Here's how the part is built. I have some questions about the finished solid (model axes, mm). A direction names the side the tool comes from. Give positions to 0.01 mm unless a question says otherwise; leave off trailing zeros. Loops run counter-clockwise (first coordinate to the right, second up) from the corner with the lowest first, then second, coordinate; pieces in that order, holes last. Notation, with made-up numbers: (-31, 32.25) - (-11, 32.25) arc R24 ccw to (-11, 69.25) - close; hole circle Ø5 at (-36, -25). An arc over 180 degrees is marked (long way). Put each result on its own line as item: value. Start each with the question number.
Autodesk Inventor part; units mm, degrees
ref_plane "YZ Plane" through (0, 0, 0) normal (1, 0, 0) x (0, 1, 0)
ref_plane "XZ Plane" through (0, 0, 0) normal (0, 1, 0) x (-1, 0, 0)
ref_plane "XY Plane" through (0, 0, 0) normal (0, 0, 1) x (1, 0, 0)
sketch "Sketch1" plane through (0, 0, 0) normal (0, 0, 1) x (1, 0, 0)
  line L0 (0, 12.6) -> (150, 12.6)
  arc A0 (150, -12.6) -> (150, 12.6) centre (150, 0) ccw
  line L1 (150, -12.6) -> (0, -12.6)
  arc A1 (0, 12.6) -> (0, -12.6) centre (0, 0) ccw
  circle A2 centre (0, 0) radius 7.5
  circle A3 centre (150, 0) radius 4.25
  dimension "d0" = 150
  dimension "d2" = 12.6
  dimension "d3" = 15
  dimension "d4" = 8.5
extrude "Extrusion1" add sketch "Sketch1" along normal blind 25
sketch "Sketch2" plane through (0, 0, 25) normal (0, 0, 1) x (1, 0, 0)
  circle A0 centre (0, 0) radius 7.5
  arc A1 (0, 12.6) -> (0, -12.6) centre (0, 0) ccw
  circle A2 centre (0, 0) radius 11
  dimension "d7" = 22
extrude "Extrusion2" cut sketch "Sketch2" against normal blind 7
sketch "Sketch4" plane through (0, 0, 25) normal (0, 0, 1) x (1, 0, 0)
  circle A0 centre (0, 0) radius 11
  circle A1 centre (20, 0) radius 1.75
  circle A2 centre (40, 0) radius 1.75
  dimension "d16" = 20
  dimension "d17" = 40
  dimension "d23" = 3.5
extrude "Extrusion3" cut sketch "Sketch4" against normal through all contours A1 | A2
sketch "Sketch5" plane through (0, 0, 25) normal (0, 0, 1) x (1, 0, 0)
  circle A0 centre (20, 0) radius 1.75
  circle A1 centre (40, 0) radius 1.75
  circle A2 centre (40, 0) radius 3
  circle A3 centre (20, 0) radius 3
  dimension "d28" = 6
extrude "Extrusion4" cut sketch "Sketch5" against normal blind 3
sketch "Sketch6" plane through (0, 0, 25) normal (0, 0, 1) x (1, 0, 0)
  line L0 (150, 12.6) -> (0, 12.6)
  arc A0 (0, 12.6) -> (0, -12.6) centre (0, 0) ccw
  line L1 (0, -12.6) -> (150, -12.6)
  arc A1 (12.1445, 12.6) -> (12.1445, -12.6) centre (0, 0) ccw
  dimension "d24" = 35
extrude "Extrusion5" add sketch "Sketch6" against normal up to surface (25 mm away)
sketch "Sketch7" plane through (0, 0, 25) normal (0, 0, 1) x (1, 0, 0)
  circle A0 centre (150, 0) radius 4.25
  arc A1 (150, -12.6) -> (150, 12.6) centre (150, 0) ccw
  circle A2 centre (150, 0) radius 7
  dimension "d30" = 14
extrude "Extrusion6" cut sketch "Sketch7" against normal blind 8
fillet "Fillet1" radius 3.5 1 edges at (-7.5, 0, 18)
sketch "Sketch8" plane through (0, 0, 25) normal (0, 0, 1) x (1, 0, 0)
  circle A0 centre (150, 0) radius 7
  line L0 (150, 12.6) -> (12.1445, 12.6)
  arc A1 (12.1445, 12.6) -> (12.1445, -12.6) centre (0, 0) ccw
  line L1 (12.1445, -12.6) -> (150, -12.6)
  line L2 (100, 12.6) -> (100, 5.75)
  line L3 (100, 5.75) -> (50, 5.75)
  line L4 (50, 5.75) -> (50, -5.75)
  line L5 (50, -5.75) -> (100, -5.75)
  line L6 (100, -5.75) -> (100, -12.6)
  dimension "d35" = 50
  dimension "d36" = 50
  dimension "d37" = 11.5
extrude "Extrusion7" cut sketch "Sketch8" against normal through all contours L2 L3 L4 L5 L6 L1 A1 L0
sketch "Sketch9" plane through (50, -5.75, 25) normal (0, -1, 0) x (1, 0, 0)
  line L0 (0, 0) -> (0, -25)
  line L1 (4.5, -8.5) -> (12.5, -8.5) construction
  line L2 (12.5, -8.5) -> (12.5, -16.5) construction
  line L3 (12.5, -16.5) -> (4.5, -16.5) construction
  line L4 (4.5, -16.5) -> (4.5, -8.5) construction
  line L5 (12.5, -16.5) -> (20.5, -16.5) construction
  line L6 (20.5, -16.5) -> (20.5, -8.5) construction
  line L7 (20.5, -8.5) -> (12.5, -8.5) construction
  line L8 (12.5, -8.5) -> (12.5, -16.5) construction
  circle A0 centre (4.5, -16.5) radius 1.75
  circle A1 centre (4, -8.5) radius 1.75
  circle A2 centre (11.5, -16.5) radius 1.75
  circle A3 centre (11, -8.5) radius 1.75
  circle A4 centre (18.5, -16.5) radius 1.75
  circle A5 centre (18, -8.5) radius 1.75
  line L9 (29.5, -8.5) -> (37.5, -8.5) construction
  line L10 (37.5, -8.5) -> (37.5, -16.5) construction
  line L11 (37.5, -16.5) -> (29.5, -16.5) construction
  line L12 (29.5, -16.5) -> (29.5, -8.5) construction
  line L13 (37.5, -16.5) -> (45.5, -16.5) construction
  line L14 (45.5, -16.5) -> (45.5, -8.5) construction
  line L15 (45.5, -8.5) -> (37.5, -8.5) construction
  line L16 (37.5, -8.5) -> (37.5, -16.5) construction
  circle A6 centre (29.5, -8.5) radius 1.75
  circle A7 centre (29, -16.5) radius 1.75
  circle A8 centre (36.5, -8.5) radius 1.75
  circle A9 centre (36, -16.5) radius 1.75
  circle A10 centre (43.5, -8.5) radius 1.75
  circle A11 centre (43, -16.5) radius 1.75
  point P0 (-50, -25)
  point P1 (0, -12.5)
  point P2 (12.5, -12.5)
  point P3 (12.5, -12.5)
  point P4 (37.5, -12.5)
  dimension "d40" = 12.5
  dimension "d41" = 8
  dimension "d42" = 0.5
  dimension "d43" = 1
  dimension "d44" = 1.5
  dimension "d45" = 2
  dimension "d46" = 2.5
  dimension "d47" = 3.5
  dimension "d48" = 25
  dimension "d49" = 0.5
  dimension "d50" = 1
  dimension "d51" = 1.5
  dimension "d52" = 2
  dimension "d53" = 2.5
extrude "Extrusion8" cut sketch "Sketch9" against normal through all
properties part number "driven arm2_2"
1) I need wall thicknesses on line 1 (Z direction, x = 79, y = 3.25); line 2 (X direction, y = 0.25, z = 18.75); line 3 (Y direction, x = 98, z = 2). Which ranges of each line are inside material? Lowest first, please.
2) Suppose I cut it at B-B on y = 1.75. Give the number of separate pieces and of enclosed holes in the cut face, plus the area to 3 significant figures.
3) Suppose I cut it at C-C on x = 61. Please give me the cut outline in (y, z), plus the area to 3 significant figures.
4) Thinking about a two-plate mould opening in X: for faces 4 (the flat face through (125, -12.6, 12)), 5 (the cylindrical face through (87.669, -0.08, 9.026)), 6 (the flat face through (50, 0, 13)), which applies, pulls with the +X half, pulls with the -X half, needs draft (parallel to the pull), parting line crosses it, or undercut?
5) Which directions (+Z, -Z, +X, -X, +Y, -Y) give clear straight access to the entire face, cutting with the end or side of a thin tool? Please do faces 1 (the cylindrical face through (80.669, -0.08, 9.026)), 2 (the flat face through (75, 5.75, 13)), 3 (the flat face through (155, 0, 17)).
6) Suppose I cut it at D-D on y = -9.75. Please give me the cut outline in (x, z), plus the area to 3 significant figures.
7) I'm going to push flat-ended pins straight in: P1, Ø12.5, axis at x = 150, y = 0, coming from the +Z side; P2, Ø7.5, axis at x = 63.5, z = 17.5, coming from the +Y side; P3, Ø3, axis at x = 93.5, z = 16.5, coming from the +Y side; P4, Ø4, axis at x = 93, z = 8.5, coming from the -Y side. Where does each tip first touch, or does it pass through?
8) Suppose I cut it at A-A on z = 4.5. Please give me the cut outline in (x, y).
Ans:
1. line 1: z = 0 to 6.75, 10.25 to 14.82, 18.18 to 25
1. line 2: x = 50 to 143, 157 to 162.6
1. line 3: y = -5.75 to 5.75
2. separate pieces: 2
2. enclosed holes: 12
2. area: 2,460 mm²
3. outline: (-5.75, 0) - (5.75, 0) - (5.75, 6.82) - (-5.75, 6.82) - close; (-5.75, 10.18) - (5.75, 10.18) - (5.75, 14.75) - (-5.75, 14.75) - close; (-5.75, 18.25) - (5.75, 18.25) - (5.75, 25) - (-5.75, 25) - close
3. area: 209 mm²
4. face 4: needs draft
4. face 5: undercut
4. face 6: pulls with the -X half
5. face 1: +Y, -Y
5. face 2: +Z, -Z, -X, +Y
5. face 3: +Z
6. outline: (100, 0) - (157.98, 0) - (157.98, 25) - (100, 25) - close
6. area: 1,450 mm²
7. P1: stops at z = 17
7. P2: stops at y = 5.75
7. P3: passes through
7. P4: stops at y = -5.75
8. outline: (50, -5.75) - (100, -5.75) - (100, -12.6) - (150, -12.6) arc R12.6 ccw to (150, 12.6) - (100, 12.6) - (100, 5.75) - (50, 5.75) - close; hole circle Ø8.5 at (150, 0)
